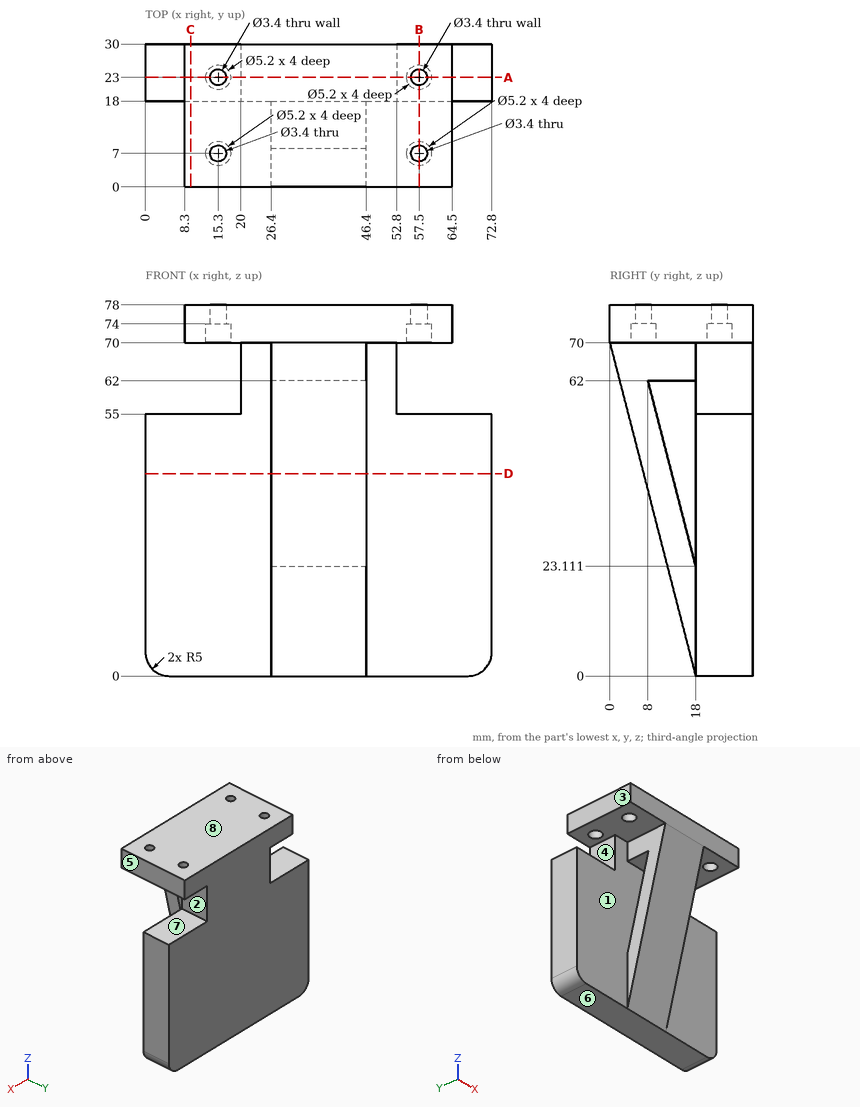
Answer from the drawing. Dimensions are ordinates in mm from the lowest x, y and z of the part. A direction names the side the tool comes from. Coordinates: 2 decimals unless noted, no trailing zeros. Loops run counter-clockwise (first coordinate to the right, second up) from the corner with the lowest first, then second, coordinate; pieces in that order, holes last.
Q1. The part is cut by section B-B on x = 57.5. Write down the section's boundary in (y, z), and give its area (3 significant figures).
Q2. The part is cut by section D-D on z = 42.5. Write down the section's boundary in (x, y).
Q3. The part is cut by section A-A on y = 23. Give the number of separate pieces and of enclosed holes in the cut face, and give its area (3 significant figures).
Q4. Consider probe 1 along Y at (x, z) = (57.5, 76.45); probe 2 along Y at (x, z) = (57.5, 71.95); probe 3 along Z at (x, y) = (9, 26.25). Determine where each line is inside the solid, lowest interval first.
Q5. Each of these flat-tipped pins is pushed along its axis until it touches: pin 1 Ø5.5 at (y, z) = (6, 47) entering from -X; pin 2 Ø10 at (x, z) = (56, 34) entering from -Y; pin 3 Ø1.5 at (x, z) = (30, 33.5) entering from -Y; pin 4 Ø2.5 at (x, y) = (15.3, 7) entering from -Z. Where does it stop, or does it pass through?
Q6. Which of the six approach directions +Z, -Z, +X, -X, +Y, -Y give full straight-line access (tool end or side, diameter ignored) to the marked faces 1, 2, 3, 4 and 5?
Q7. The mould has two halves that part along Z. Classify the marked faces 6, 7 and 8: +Z half, -Z half, draft (parallel to the pull), parting line (faces both ways), or undercut.
Q8. The part is cut by section C-C on x = 9.5. Write down the section's boundary in (y, z), and give its area (3 significant figures).
Results below:
1. outline: (0, 70) - (4.4, 70) - (4.4, 74) - (5.3, 74) - (5.3, 78) - (0, 78) - close; (8.7, 74) - (9.6, 74) - (9.6, 70) - (20.4, 70) - (20.4, 74) - (21.3, 74) - (21.3, 78) - (8.7, 78) - close; (18, 0) - (30, 0) - (30, 55) - (18, 55) - close; (24.7, 74) - (25.6, 74) - (25.6, 70) - (30, 70) - (30, 78) - (24.7, 78) - close
1. area: 831 mm2
2. outline: (0, 18) - (72.8, 18) - (72.8, 30) - (0, 30) - close; (26.4, 7.07) - (46.4, 7.07) - (46.4, 13.01) - (26.4, 13.01) - close
3. separate pieces: 3
3. enclosed holes: 0
3. area: 4,870 mm2
4. probe 1: y = 0 to 5.3, 8.7 to 21.3, 24.7 to 30
4. probe 2: y = 0 to 4.4, 9.6 to 20.4, 25.6 to 30
4. probe 3: z = 0 to 55, 70 to 78
5. pin 1: stops at x = 26.4
5. pin 2: stops at y = 18
5. pin 3: stops at y = 9.19
5. pin 4: passes through
6. face 1: none
6. face 2: +X, +Y, -Y
6. face 3: +Z, -X, +Y, -Y
6. face 4: -X, +Y, -Y
6. face 5: +Z, +X, +Y, -Y
7. face 6: -Z half
7. face 7: undercut
7. face 8: +Z half
8. outline: (0, 70) - (30, 70) - (30, 78) - (0, 78) - close; (18, 0) - (30, 0) - (30, 55) - (18, 55) - close
8. area: 900 mm2
